```python
from build123d import *

# Parameters (mm, degrees)
SKETCH1_W           = 57.4
SKETCH1_H           = 33
BOSS_EXTRUDE1_DEPTH = 7
SHELL3_T            = -2
SKETCH2_R           = 1.65
CUT_EXTRUDE1_DEPTH  = 67.398493959
SKETCH3_W           = 40.5
SKETCH3_H           = 3.2
CUT_EXTRUDE2_DEPTH  = 67.398493959
SKETCH4_W           = 2
SKETCH4_H           = 10
CUT_EXTRUDE3_DEPTH  = 5
SKETCH5_W           = 57.4
SKETCH5_H           = 2
BOSS_EXTRUDE2_DEPTH = 5
CUT_EXTRUDE4_REACH  = 69.289
SKETCH6_R           = 1.15
FILLET1_R           = 2


with BuildPart() as part:
    # Sketch1 → Boss-Extrude1 (new body)
    with BuildSketch(Plane(origin=(0, 0, 0), x_dir=(1, 0, 0), z_dir=(0, 1, 0))):
        with Locations((28.7, 16.5)):
            Rectangle(SKETCH1_W, SKETCH1_H)
    extrude(amount=BOSS_EXTRUDE1_DEPTH)

    # Shell3
    shell3_openings = [part.faces().sort_by_distance(p)[0] for p in [
        (28.7, 7, -16.5),
    ]]
    offset(amount=SHELL3_T, openings=shell3_openings, kind=Kind.INTERSECTION)

    # Sketch2 → Cut-Extrude1 (cut, through all)
    with BuildSketch(Plane(origin=(0, 2, 0), x_dir=(1, 0, 0), z_dir=(0, 1, 0))):
        with Locations(Location((4.5, 28.3, 0), (0, 0, 270))):
            Circle(SKETCH2_R)
        with Locations(Location((51.5, 28.3, 0), (0, 0, 270))):
            Circle(SKETCH2_R)
        with Locations(Location((4.5, 4.7, 0), (0, 0, 270))):
            Circle(SKETCH2_R)
        with Locations(Location((51.5, 4.7, 0), (0, 0, 270))):
            Circle(SKETCH2_R)
    extrude(amount=-CUT_EXTRUDE1_DEPTH, mode=Mode.SUBTRACT)

    # Sketch3 → Cut-Extrude2 (cut, through all)
    with BuildSketch(Plane(origin=(0, 2, 0), x_dir=(1, 0, 0), z_dir=(0, 1, 0))):
        with Locations((27.25, 29.4)):
            Rectangle(SKETCH3_W, SKETCH3_H)
        with Locations((27.25, 3.6)):
            Rectangle(SKETCH3_W, SKETCH3_H)
    extrude(amount=-CUT_EXTRUDE2_DEPTH, mode=Mode.SUBTRACT)

    # Sketch4 → Cut-Extrude3 (cut)
    with BuildSketch(Plane(origin=(0, 7, 0), x_dir=(1, 0, 0), z_dir=(0, 1, 0))):
        with Locations((56.4, 16.5)):
            Rectangle(SKETCH4_W, SKETCH4_H)
    extrude(amount=-CUT_EXTRUDE3_DEPTH, mode=Mode.SUBTRACT)

    # Sketch5 → Boss-Extrude2 (add)
    with BuildSketch(Plane(origin=(0, 7, 0), x_dir=(1, 0, 0), z_dir=(0, 1, 0))):
        with Locations((28.7, 32)):
            Rectangle(SKETCH5_W, SKETCH5_H)
    extrude(amount=BOSS_EXTRUDE2_DEPTH)

    # Sketch6 → Cut-Extrude4 (cut, up to next)
    with BuildSketch(Plane(origin=(0, 0, -33), x_dir=(-1, 0, 0), z_dir=(0, 0, -1)), mode=Mode.PRIVATE) as cut_extrude4_sk1:
        with Locations((-38.7, 10)):
            Circle(SKETCH6_R)
    cut_extrude4_tool1 = extrude(cut_extrude4_sk1.sketch, amount=-CUT_EXTRUDE4_REACH, mode=Mode.PRIVATE) & part.part
    # Sketch6 → Cut-Extrude4 (cut, up to next)
    with BuildSketch(Plane(origin=(0, 0, -33), x_dir=(-1, 0, 0), z_dir=(0, 0, -1)), mode=Mode.PRIVATE) as cut_extrude4_sk2:
        with Locations((-18.7, 10)):
            Circle(SKETCH6_R)
    cut_extrude4_tool2 = extrude(cut_extrude4_sk2.sketch, amount=-CUT_EXTRUDE4_REACH, mode=Mode.PRIVATE) & part.part
    add(cut_extrude4_tool1.solids().sort_by_distance((38.7, 10, -33))[0], mode=Mode.SUBTRACT)
    add(cut_extrude4_tool2.solids().sort_by_distance((18.7, 10, -33))[0], mode=Mode.SUBTRACT)

    # Fillet1
    fillet1_edges = [part.edges().sort_by_distance(p)[0] for p in [
        (57.4, 3.5, 0),
        (0, 3.5, 0),
    ]]
    fillet(fillet1_edges, radius=FILLET1_R)


solid = part.part
```
Geometry: final body of the model. Coordinates: model frame, mm. A direction names the side the tool comes from. Coordinates: 2 decimals unless noted, no trailing zeros. Order: outer loops, then holes, each group sorted by start corner. A loop starts at its lowest first (then second) coordinate and runs counter-clockwise, first axis right, second up. Notation, with made-up numbers: (29, -34.5) - (44, -34.5) arc R23 ccw to (44, -7.5) - close; hole circle Ø5 at (-13, 75.5). An arc over 180 degrees is marked (long way). Return JSON: item names as keys, results as strings. Group by question number.
1. Cut plane A-A (x = 51.5). Output: boundary loops of the cut face in (y, z), plus the area to 3 significant figures.
2. Cut plane C-C (y = 3.75). Output: boundary loops of the cut face in (x, z), plus the area to 3 significant figures.
3. Material intervals for line 1 along X through (y, z) = (1, -4.7); line 2 along Z through (x, y) = (53, 6); line 3 along Y through (x, z) = (11.5, -20.5), sorted ascending. Write a range as [from, to].
4. Pull-direction query (Y, two-part tool) for faces 4 (the face through (19.61, 9.3, -32.01)), 5 (the face through (28, 0, -17)), 6 (the face through (38.17, 8.98, -32.01)), 7 (the face through (55.4, 4, -26)); classes: pulls with the +Y half, pulls with the -Y half, needs draft (parallel to the pull), parting line crosses it, or undercut.
5. Cut plane B-B (x = 38.7). Output: boundary loops of the cut face in (y, z), plus the area to 3 significant figures.
6. Set-up query: faces 1 (the face through (47.5, 1, -4)), 2 (the face through (55.4, 4, -7)), 3 (the face through (56, 5, -11.5)). Return all of +Z, -Z, +X, -X, +Y, -Y with unobstructed straight access to the full face (end or side cutting, diameter ignored); none if empty.
7. Pin query (flat end, axial travel): pin 1 (6 mm diameter, centred on x = 50.5, y = 8, fed in from +Z); pin 2 (2 mm diameter, centred on x = 38.5, y = 9.5, fed in from +Z); pin 3 (3 mm diameter, centred on x = 38, z = -15.5, fed in from +Y). Return the tip coordinate at first contact, or that it passes through.
8. Cut plane D-D (z = -23.5). Output: boundary loops of the cut face in (x, y), plus the area to 3 significant figures.
Resolved:
{
 "1": {"outline": "(0, -33) - (12, -33) - (12, -31) - (2, -31) - (2, -29.95) - (0, -29.95) - close; (0, -26.65) - (2, -26.65) - (2, -6.35) - (0, -6.35) - close; (0, -3.05) - (2, -3.05) - (2, -2) - (7, -2) - (7, 0) - (0, 0) - close", "area": "82.8 mm²"},
 "2": {"outline": "(0, -33) - (57.4, -33) - (57.4, -21.5) - (55.4, -21.5) - (55.4, -31) - (2, -31) - (2, -2) - (55.4, -2) - (55.4, -11.5) - (57.4, -11.5) - (57.4, -2) arc R2 ccw to (55.4, 0) - (2, 0) arc R2 ccw to (0, -2) - close", "area": "324 mm²"},
 "3": {"line 1": "x = [0, 2.85], [6.15, 7], [47.5, 49.85], [53.15, 57.4]", "line 2": "z = [-33, -31], [-2, 0]", "line 3": "y = [0, 2]"},
 "4": {"face 4": "undercut", "face 5": "pulls with the -Y half", "face 6": "undercut", "face 7": "needs draft"},
 "5": {"outline": "(0, -33) - (8.85, -33) - (8.85, -31) - (0, -31) - close; (0, -27.8) - (2, -27.8) - (2, -5.2) - (0, -5.2) - close; (0, -2) - (7, -2) - (7, 0) - (0, 0) - close; (11.15, -33) - (12, -33) - (12, -31) - (11.15, -31) - close", "area": "78.6 mm²"},
 "6": {"face 1": "+Y, -Y", "face 2": "+Y", "face 3": "+X, +Y"},
 "7": {"pin 1": "stops at z = 0", "pin 2": "stops at z = -31", "pin 3": "stops at y = 2"},
 "8": {"outline": "(0, 0) - (57.4, 0) - (57.4, 7) - (55.4, 7) - (55.4, 2) - (2, 2) - (2, 7) - (0, 7) - close", "area": "135 mm²"}
}
